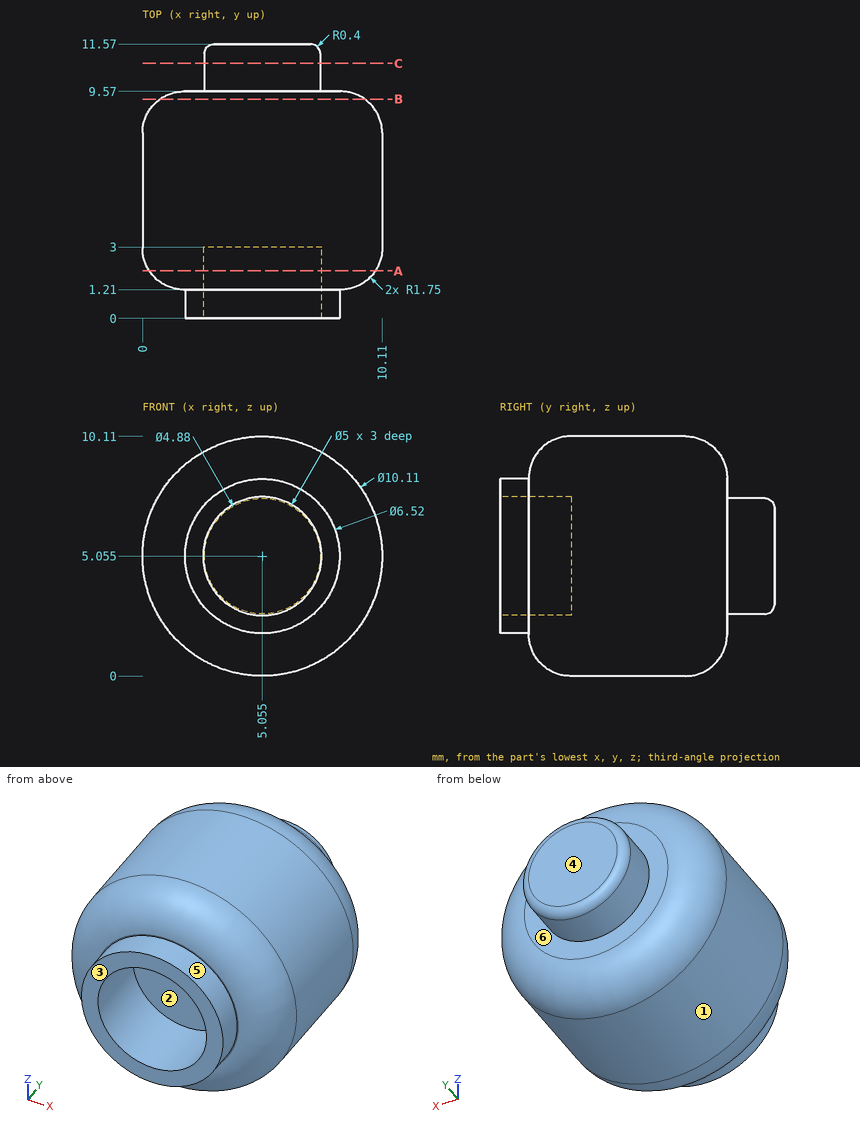
Input: dimensioned drawing with shaded views. Units: mm. Origin: part minimum x, y, z. A direction names the side the tool comes from. Give positions to 0.01 mm unless a question says otherwise; leave off trailing zeros. Loops run counter-clockwise (first coordinate to the right, second up) from the corner with the lowest first, then second, coordinate; pieces in that order, holes last. Notation, with made-up numbers: (-2, -33.5) -> (36, -33.5) arc R15 ccw to (36, -27.5) -> close; hole circle Ø1 at (-3, 27.25). An arc over 180 degrees is marked (long way). Return JSON: item names as keys, results as strings.
Item 1: Section C-C, the plane y = 10.75. Output: boundary loops of the cut face in (x, z) (3 decimals).
Filled in:
{"outline": "circle Ø4.88 at (5.055, 5.055)"}
Item 2: Mould query, pull axis X, two halves, no side actions, for the marked faces 1, 2 and 3. Classes: released by +X, released by -X, zero draft, split by the parting line, or undercut.
Filled in:
{"face 1": "split by the parting line", "face 2": "undercut", "face 3": "zero draft"}
Item 3: Access query for the marked faces 4, 5 and 6. Directions: +Z, -Z, +X, -X, +Y, -Y. A direction counts if a zero-diameter tool reaches every point of the face in a straight line with its end or side. Return the directions, or none.
Filled in:
{"face 4": "+Z, -Z, +X, -X, +Y", "face 5": "-Y", "face 6": "+Y"}
Item 4: Section A-A, the plane y = 2. Output: boundary loops of the cut face in (x, z) (3 decimals), plus the area to 3 significant figures.
Filled in:
{"outline": "circle Ø9.536 at (5.055, 5.055); hole circle Ø5 at (5.055, 5.055)", "area": "51.8 mm^2"}
Item 5: Pin query (flat end, axial travel): P1, Ø1.5, axis at x = 5, z = 4, coming from the -Y side; P2, Ø3, axis at x = 2.5, y = 4, coming from the -Z side; P3, Ø1, axis at x = 2, y = 7.5, coming from the +Z side. Return the tip coordinate at first contact, or that it passes through.
Filled in:
{"P1": "y = 3", "P2": "z = 0.11", "P3": "z = 9.42"}
Item 6: Section B-B, the plane y = 9.25. Output: boundary loops of the cut face in (x, z) (3 decimals).
Filled in:
{"outline": "circle Ø8.628 at (5.055, 5.055)"}
Item 7: Line query: line 1 (Y direction, x = 4.75, z = 4.5); line 2 (Z direction, x = 6.5, y = 7.25); line 3 (X direction, y = 4.25, z = 8.5). Output: solid intervals per line, ascending.
Filled in:
{"line 1": "3 to 11.57", "line 2": "0.21 to 9.9", "line 3": "1.36 to 8.75"}
